from build123d import *

# Parameters (mm, degrees)
SALIENTE_EXTRUIR1_DEPTH = 437.896
CROQUIS2_R              = 3.999992
CORTAR_EXTRUIR1_DEPTH   = 4.064
CROQUIS3_R              = 2.5
CORTAR_EXTRUIR2_DEPTH   = 1.499997


with BuildPart() as part:
    # Croquis1 → Saliente-Extruir1 (new body)
    with BuildSketch(Plane.XY):
        Polygon((0, 0), (0, 50.8), (1.499997, 50.8), (1.499997, 1.499997), (50.8, 1.499997), (50.8, 0), align=None)
    extrude(amount=SALIENTE_EXTRUIR1_DEPTH)

    # Croquis2 → Cortar-Extruir1 (cut)
    with BuildSketch(Plane.ZY):
        with Locations((266.948, 25.4)):
            Circle(CROQUIS2_R)
        with Locations((362.948, 25.4)):
            Circle(CROQUIS2_R)
        with Locations((74.948, 25.4)):
            Circle(CROQUIS2_R)
        with Locations((170.948, 25.4)):
            Circle(CROQUIS2_R)
    extrude(amount=-CORTAR_EXTRUIR1_DEPTH, mode=Mode.SUBTRACT)

    # Croquis3 → Cortar-Extruir2 (cut)
    with BuildSketch(Plane.ZY):
        with Locations((18.948, 29.8)):
            Circle(CROQUIS3_R)
        with Locations((118.948, 29.8)):
            Circle(CROQUIS3_R)
        with Locations((218.948, 29.8)):
            Circle(CROQUIS3_R)
        with Locations((318.948, 29.8)):
            Circle(CROQUIS3_R)
        with Locations((418.948, 29.8)):
            Circle(CROQUIS3_R)
        with Locations((18.948, 6.8)):
            Circle(CROQUIS3_R)
        with Locations((218.948, 6.8)):
            Circle(CROQUIS3_R)
        with Locations((118.948, 6.8)):
            Circle(CROQUIS3_R)
        with Locations((318.948, 6.8)):
            Circle(CROQUIS3_R)
        with Locations((418.948, 6.8)):
            Circle(CROQUIS3_R)
    extrude(amount=-CORTAR_EXTRUIR2_DEPTH, mode=Mode.SUBTRACT)


solid = part.part
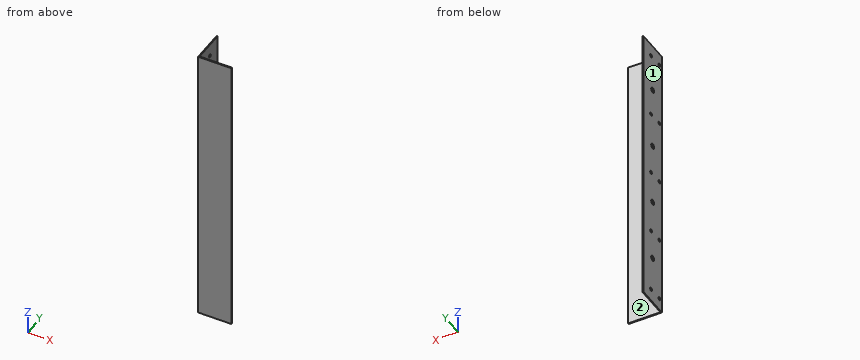
Design review of the part built by this model. Coordinates are the model's own, in mm. Face numbers are marked on the shaded views. A direction names the side the tool comes from. Round coordinates to 2 decimals unless told otherwise and drop trailing zeros. Write each loop counter-clockwise with the first axis right and the second up, starting at its lowest first coordinate (ties: lowest second). Pieces come first, ordered by that corner, then holes.
Item 1: Wall thickness on L1, parallel to Y at x = 37, z = 48.5: over which ranges is the line inside the solid? List them lowest first.
Item 2: Consider section B-B on x = 33.5. Give the boundary of the cut face in (y, z).
Item 3: Consider section A-A on z = 183. Give the boundary of the cut face in (x, y), and give its area (3 significant figures).
Item 4: For the marked faces 1 and 2, list the 3-axis set-ups (+Z, -Z, +X, -X, +Y, -Y) from which the entire face can be reached by the end or side of a thin tool; tool diameter is ignored.
Item 5: For pin 1 Ø1.5 at (x, z) = (27, 331) entering from +Y; pin 2 Ø6 at (y, z) = (6.8, 318.948) entering from +X, all flat-tipped, find the tip position at first contact; note any pin that passes through.
Check values:
1. L1: y = 0 to 1.5
2. outline: (0, 0) - (1.5, 0) - (1.5, 437.9) - (0, 437.9) - close
3. outline: (0, 0) - (50.8, 0) - (50.8, 1.5) - (1.5, 1.5) - (1.5, 50.8) - (0, 50.8) - close
3. area: 150 mm2
4. face 1: +Z, -Z, -X, +Y, -Y
4. face 2: +Z, -Z, +X, +Y
5. pin 1: stops at y = 1.5
5. pin 2: stops at x = 1.5
